Design review of the part built by this model. Coordinates are the model's own, in mm. A direction names the side the tool comes from. Round coordinates to 2 decimals unless told otherwise and drop trailing zeros. Loops run counter-clockwise (first coordinate to the right, second up) from the corner with the lowest first, then second, coordinate; pieces in that order, holes last. Notation, with made-up numbers: (27, 35.5) - (78, 35.5) arc R4 ccw to (78, 40.5) - close; hole circle Ø1 at (57.5, 89.5). An arc over 180 degrees is marked (long way). Answer as CSV lines item,"result". Start each with the question number.
(1) For faces 4 (the cylindrical face through (-3.457, -54.517, 29.073)), 5 (the flat face through (-25.3, -33.5, 10.7)), 6 (the flat face through (-3, -34, 13.143)), list the 3-axis set-ups (+Z, -Z, +X, -X, +Y, -Y) from which the entire face can be reached by the end or side of a thin tool; tool diameter is ignored.
(2) Mouldability with a two-part tool opening along Z and no side actions: class faces 1 (the cylindrical face through (-32.79, -54.81, 29.07)), 2 (the flat face through (-33, -34, 13.143)), 3 (the cylindrical face through (-21.685, -33.524, 18.1)) as released by +Z, released by -Z, zero draft, split by the parting line, or undercut.
(3) Wall thickness on L1, parallel to X at y = -56.5, z = 31.75; L2, parallel to Y at x = -33, z = 24.5; L3, parallel to X at y = -11, z = 25: over which ranges is each line inside the solid? List them lowest first.
(4) Consider section A-A (x = -20.5). Give the boundary of the cut face in (y, z).
(5) Consider section C-C (y = -52). Give the boundary of the cut face in (x, z).
(6) For P1, Ø11, axis at x = -1.5, y = -32, coming from the -Z side; P2, Ø10, axis at x = -6, y = -13.5, coming from the -Z side; P3, Ø13, axis at x = -17.72, z = 21.14, coming from the -Y side; P4, Ø3.5, axis at x = -31.72, y = -56.5, coming from the +Z side, all flat-tipped, find the tip position at first contact; note any pin that passes through.
(7) Consider section B-B (z = 28.25). Give the boundary of the cut face in (x, y).
from build123d import *

# Parameters (mm, degrees)
F0_R     = 5
F1_DEPTH = 68
F3_D     = 4
F3_DEPTH = 10
F3_TIP   = 1.2017212381


with BuildPart() as f1:
    # F0 (on Front) → F1 (new body)
    with BuildSketch(Plane.XZ):
        Polygon((2.2830869555, 34.1427520012), (-37.7169130445, 34.1427520012), (-37.7169130445, 13.1427520012), (-27.8874205338, 13.1427520012), (-22.5867759436, 8.1427520012), (-12.8470501453, 8.1427520012), (-7.5464055551, 13.1427520012), (2.2830869555, 13.1427520012), align=None)
        with Locations((-17.7169130445, 21.1427520012)):
            Circle(F0_R, mode=Mode.SUBTRACT)
    extrude(amount=F1_DEPTH)

    # F3
    with Locations(Plane.XY.offset(34.1427520012)):
        with Locations((-31.7169130445, -11.5), (-31.7169130445, -56.5), (-3.7169130445, -11.5), (-3.7169130445, -56.5)):
            Hole(F3_D / 2, depth=F3_DEPTH)
            with Locations((0, 0, -(F3_DEPTH + F3_TIP / 2))):  # 118° drill point
                Cone(0, F3_D / 2, F3_TIP, mode=Mode.SUBTRACT)


solid = f1.part
Determined:
1,face 4,"+Z"
1,face 5,"-Z, -X, +Y, -Y"
1,face 6,"-Z, +X, +Y, -Y"
2,face 1,"zero draft"
2,face 2,"released by -Z"
2,face 3,"undercut"
3,L1,"x = -37.72 to -33.72, -29.72 to -5.72, -1.72 to 2.28"
3,L2,"y = -68 to -58.03, -54.97 to -13.03, -9.97 to 0"
3,L3,"x = -37.72 to -33.65, -29.78 to -20.9, -14.54 to -5.65, -1.78 to 2.28"
4,outline,"(-68, 8.14) - (0, 8.14) - (0, 16.99) - (-68, 16.99) - close; (-68, 25.3) - (0, 25.3) - (0, 34.14) - (-68, 34.14) - close"
5,outline,"(-37.72, 13.14) - (-27.89, 13.14) - (-22.59, 8.14) - (-12.85, 8.14) - (-7.55, 13.14) - (2.28, 13.14) - (2.28, 34.14) - (-37.72, 34.14) - close; hole circle Ø10 at (-17.72, 21.14)"
6,P1,"stops at z = 13.14"
6,P2,"stops at z = 9.89"
6,P3,"stops at y = -68"
6,P4,"stops at z = 23.99"
7,outline,"(-37.72, -68) - (2.28, -68) - (2.28, 0) - (-37.72, 0) - close; hole circle Ø4 at (-31.72, -56.5); hole circle Ø4 at (-31.72, -11.5); hole circle Ø4 at (-3.72, -56.5); hole circle Ø4 at (-3.72, -11.5)"
